Check sheet for the modelled part. Datum: model origin and axes. Units: mm. Face numbers are marked on the shaded views. A direction names the side the tool comes from. Round coordinates to 2 decimals unless told otherwise and drop trailing zeros. Loops run counter-clockwise (first coordinate to the right, second up) from the corner with the lowest first, then second, coordinate; pieces in that order, holes last. Notation, with made-up numbers: (37.25, -32) -> (74.25, -32) arc R17 ccw to (74.25, -12) -> close; hole circle Ø5 at (34, 17.25). An arc over 180 degrees is marked (long way). One line per item, written item: value. Start each with the question number.
1. Cross-section at B-B on y = -69.5. Record the cut outline in (x, z).
2. Set-up check for the marked faces 1 and 2: record each of +Z, -Z, +X, -X, +Y, -Y from which the full face is reachable in a straight line by a thin tool's end or side.
3. Cross-section at A-A on x = 30.5. Record the cut outline in (y, z), then the cut area to 3 significant figures.
4. Material ranges on L1, parallel to Z at x = 44, y = -90; L2, parallel to Y at x = -1, z = 26; L3, parallel to Z at x = 15.5, y = 8.5, recorded low to high.
5. Go/stop test with flat-tipped pins: pin 1 (3 mm diameter, centred on y = -57, z = 27, fed in from -X); pin 2 (1 mm diameter, centred on x = 36.5, y = -9, fed in from +Z). Record where each tip stops, or that it passes through.
from build123d import *

# Parameters (mm, degrees)
F0_W     = 100
F0_H     = 200
F1_DEPTH = 25
F2_W     = 100
F2_H     = 10.1669974625
F3_DEPTH = 100
F5_DEPTH = 200


with BuildPart() as f1:
    # F0 (on Top) → F1 (new body)
    with BuildSketch(Plane.XY):
        Rectangle(F0_W, F0_H)
    extrude(amount=F1_DEPTH)

    # F2 (on face) → F3 (join)
    with BuildSketch(Plane.YZ.offset(50)):
        with Locations((50, 30.0834987313)):
            Rectangle(F2_W, F2_H)
    extrude(amount=-F3_DEPTH)

    # F4 (on face) → F5 (cut)
    with BuildSketch(Plane.YZ.offset(50)):
        Polygon((0, 35.1669974625), (0, 25), (11.165715754, 35.1669974625), align=None)
    extrude(amount=-F5_DEPTH, mode=Mode.SUBTRACT)


solid = f1.part
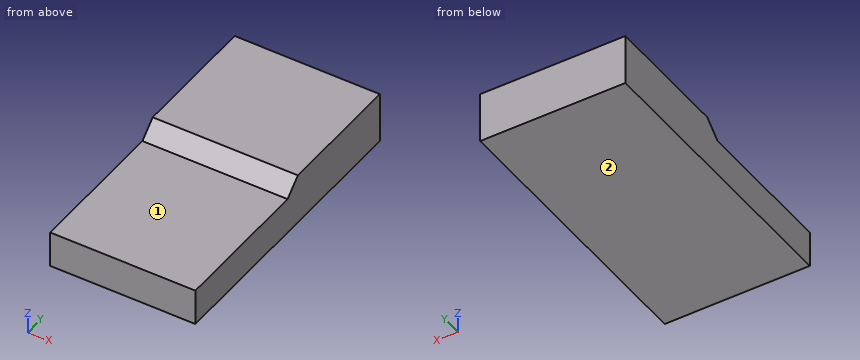
Taken from the geometry:
1. outline: (-50, 0) -> (50, 0) -> (50, 25) -> (-50, 25) -> close
2. face 1: +Z, +X, -X, -Y
2. face 2: -Z, +X, -X, +Y, -Y
3. outline: (-100, 0) -> (100, 0) -> (100, 35.17) -> (11.17, 35.17) -> (0, 25) -> (-100, 25) -> close
3. area: 5,960 mm2
4. L1: z = 0 to 25
4. L2: y = 1.1 to 100
4. L3: z = 0 to 32.74
5. pin 1: passes through
5. pin 2: stops at z = 25
